Here's how the part is built. I have some questions about the finished solid (model axes, mm). Coordinates: 2 decimals unless noted, no trailing zeros. Write each loop counter-clockwise with the first axis right and the second up, starting at its lowest first coordinate (ties: lowest second). Pieces come first, ordered by that corner, then holes. Notation, with made-up numbers: (88, -20.75) -> (95, -20.75) arc R21 ccw to (95, 4.25) -> close; hole circle Ø11 at (37, -20.75). An arc over 180 degrees is marked (long way). Use a Markdown table: item, result. Add a question column.
Item 1: Imagine slicing it at B-B, the plane x = -202.5. Count the separate pieces of the cut face and the enclosed holes in it, and give its area (3 significant figures).
Item 2: Will these pins go through, and if not, where does the flat tip stop? pin 1 Ø10 at (x, z) = (-202.3, 74.61) entering from +Y; pin 2 Ø12.5 at (x, z) = (-116.17, -82) entering from -Y.
Item 3: Imagine slicing it at A-A, the plane z = -82. Write out the boundary of the cut face in (x, y).
Item 4: If I drill on line 1 along Z through (x, y) = (-202.5, 9); line 2 along X through (y, z) = (11, -82.5), over which ranges is the centre line in solid material (lowest first)? Write a range as from..to.
```python
from build123d import *

# Parameters (mm, degrees)
SKETCH1_W                                            = 465
SKETCH1_H                                            = 300
BOSS_EXTRUDE1_DEPTH                                  = 12
CSK_FOR_M10_COUNTERSUNK_FLAT_HEAD_SCREW1_D           = 11
CSK_FOR_M10_COUNTERSUNK_FLAT_HEAD_SCREW1_DEPTH       = 20.003
CSK_FOR_M10_COUNTERSUNK_FLAT_HEAD_SCREW1_CSINK_D     = 20
CSK_FOR_M10_COUNTERSUNK_FLAT_HEAD_SCREW1_CSINK_ANGLE = 90
CSK_FOR_M10_COUNTERSUNK_FLAT_HEAD_SCREW1_TIP         = 3.304733405


with BuildPart() as part:
    # Sketch1 → Boss-Extrude1 (new body)
    with BuildSketch(Plane(origin=(0, 0, 0), x_dir=(1, 0, 0), z_dir=(0, 1, 0))):
        Rectangle(SKETCH1_W, SKETCH1_H)
    extrude(amount=BOSS_EXTRUDE1_DEPTH)

    # CSK for M10 Countersunk Flat Head Screw1
    with Locations(Plane(origin=(0, 0, 0), x_dir=(-1, 0, 0), z_dir=(0, -1, 0))):
        with Locations((116.169058485, -74.612719009), (202.304435362, -74.612719009), (202.5, 82), (116.169058485, 82)):
            CounterSinkHole(CSK_FOR_M10_COUNTERSUNK_FLAT_HEAD_SCREW1_D / 2, CSK_FOR_M10_COUNTERSUNK_FLAT_HEAD_SCREW1_CSINK_D / 2, depth=CSK_FOR_M10_COUNTERSUNK_FLAT_HEAD_SCREW1_DEPTH, counter_sink_angle=CSK_FOR_M10_COUNTERSUNK_FLAT_HEAD_SCREW1_CSINK_ANGLE)
            with Locations((0, 0, -(CSK_FOR_M10_COUNTERSUNK_FLAT_HEAD_SCREW1_DEPTH + CSK_FOR_M10_COUNTERSUNK_FLAT_HEAD_SCREW1_TIP / 2))):  # 118° drill point
                Cone(0, CSK_FOR_M10_COUNTERSUNK_FLAT_HEAD_SCREW1_D / 2, CSK_FOR_M10_COUNTERSUNK_FLAT_HEAD_SCREW1_TIP, mode=Mode.SUBTRACT)


solid = part.part
```
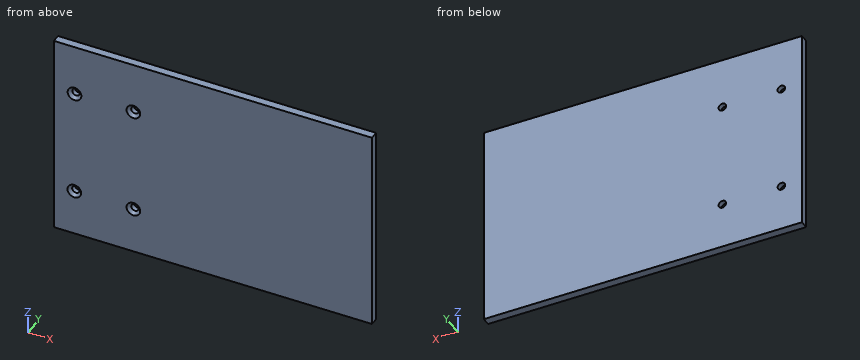
Ans:
| question | item | result |
|---|---|---|
| 1 | separate pieces | 3 |
| 1 | enclosed holes | 0 |
| 1 | area | 3,300 mm^2 |
| 2 | pin 1 | passes through |
| 2 | pin 2 | stops at y = 3.75 |
| 3 | outline | (-232.5, 0) -> (-212.5, 0) -> (-208, 4.5) -> (-208, 12) -> (-232.5, 12) -> close; (-197, 4.5) -> (-192.5, 0) -> (-126.17, 0) -> (-121.67, 4.5) -> (-121.67, 12) -> (-197, 12) -> close; (-110.67, 4.5) -> (-106.17, 0) -> (232.5, 0) -> (232.5, 12) -> (-110.67, 12) -> close |
| 4 | line 1 | z = -150..-87.5, -76.5..69.12, 80.11..150 |
| 4 | line 2 | x = -232.5..-207.98, -197.02..-121.65, -110.69..232.5 |
